```python
from build123d import *

# Parameters (mm, degrees)
F1_DEPTH = 88.9
F3_D     = 19.05
F5_D     = 4.7625


# Not quite as in the source:
# - a feature names something its author has since deleted; it is built from what else it names


with BuildPart() as f1:
    # F0 (on Top) → F1 (new body)
    with BuildSketch(Plane.XY):
        Polygon((10.538799933, 10.6713908286), (-57.7562613184, 10.6713908286), (-65.16550908, 2.3876), (-62.4960911285, 0), (-56.1460911285, 7.0995158286), (8.9414088715, 7.0995158286), (15.2914088715, 0), (17.9537273073, 2.38125), align=None)
    extrude(amount=F1_DEPTH)

    # F3 (through all)
    with Locations(Plane(origin=(0, 10.6713908286, 0), x_dir=(-1, 0, 0), z_dir=(0, 1, 0))):
        with Locations((22.8085911285, 60.325), (23.6087306927, 28.575)):
            Hole(F3_D / 2)

    # F5 (through all)
    with Locations(Plane(origin=(0, 10.6713908286, 0), x_dir=(-1, 0, 0), z_dir=(0, 1, 0))):
        with Locations((-2.5914088715, 82.55), (29.9205911285, 82.55), (29.9205911285, 13.97), (-2.5914088715, 13.97), (48.2085911285, 11.0998), (48.2085911285, 77.7748), (6.9335911285, 77.7748), (6.9335911285, 11.0998)):
            Hole(F5_D / 2)


solid = f1.part
```
Here's how the part is built. I have some questions about the finished solid (model axes, mm). A direction names the side the tool comes from. Coordinates: 2 decimals unless noted, no trailing zeros. Write each loop counter-clockwise with the first axis right and the second up, starting at its lowest first coordinate (ties: lowest second). Pieces come first, ordered by that corner, then holes. Notation, with made-up numbers: (-6, 59) - (44, 59) arc R17 cw to (44, 76) - close; hole circle Ø3 at (73, 75.5). An arc over 180 degrees is marked (long way). One line per item, written item: value.
1) I'm going to push flat-ended pins straight in: P1, Ø5.5, axis at x = 2.59, z = 82.55, coming from the -Y side; P2, Ø3, axis at x = -48.21, z = 11.1, coming from the +Y side; P3, Ø1, axis at y = 6, z = 27, coming from the -X side; P4, Ø1, axis at y = 5.5, z = 49, coming from the +X side. Where does each tip first touch, or does it pass through?
Model answer:
P1: stops at y = 7.1
P2: passes through
P3: stops at x = -62.38
P4: stops at x = 15.61
2) On a 3-axis mill with a long thin cutter (end or side, diameter ignored), from which of +Z, -Z, +X, -X, +Y, -Y can I reach the whole of each face in a straight line? I mean faces 1 (the cylindrical face through (2.075, 8.86, 80.225)), 2 (the flat face through (-24, 7.1, 44)). Say none if no direction works.
Model answer:
face 1: +Y, -Y
face 2: +Z, -Z, -Y
3) Suppose I cut it at D-D on y = 9. State how many separate pieces and enclosed holes the cut face has, and give its area (3 significant figures).
Model answer:
separate pieces: 1
enclosed holes: 10
area: 5,620 mm²
4) Suppose I cut it at C-C on z = 42. Write out the boundary of the cut face in (x, y).
Model answer:
outline: (-65.17, 2.39) - (-62.5, 0) - (-56.15, 7.1) - (8.94, 7.1) - (15.29, 0) - (17.95, 2.38) - (10.54, 10.67) - (-57.76, 10.67) - close
5) I need wall thicknesses on line 1 along Z through (x, y) = (3.5, 8); line 2 along Y through (x, z) = (0, 57); line 3 along X through (y, z) = (6.75, 47). Which ranges of each line are inside material? Lowest first, please.
Model answer:
line 1: z = 0 to 11.77, 16.17 to 80.35, 84.75 to 88.9
line 2: y = 7.1 to 10.67
line 3: x = -61.26 to -56.46, 9.25 to 14.05
6) Suppose I cut it at B-B on x = -48. Write out the boundary of the cut face in (y, z), and give its area (3 significant figures).
Model answer:
outline: (7.1, 0) - (10.67, 0) - (10.67, 8.73) - (7.1, 8.73) - close; (7.1, 13.47) - (10.67, 13.47) - (10.67, 75.4) - (7.1, 75.4) - close; (7.1, 80.15) - (10.67, 80.15) - (10.67, 88.9) - (7.1, 88.9) - close
area: 284 mm²
7) Suppose I cut it at A-A on z = 82.55. Write out the boundary of the cut face in (x, y), and give its area (3 significant figures).
Model answer:
outline: (-65.17, 2.39) - (-62.5, 0) - (-56.15, 7.1) - (-32.3, 7.1) - (-32.3, 10.67) - (-57.76, 10.67) - close; (-27.54, 7.1) - (0.21, 7.1) - (0.21, 10.67) - (-27.54, 10.67) - close; (4.97, 7.1) - (8.94, 7.1) - (15.29, 0) - (17.95, 2.38) - (10.54, 10.67) - (4.97, 10.67) - close
area: 278 mm²
8) We'd pull the mould along X, two halves only. Please class faces 3 (the flat face through (14.298, 6.468, 43.828)), 4 (the flat face through (-63.85, 1.21, 43.83)), 5 (the flat face through (-59.366, 3.5, 43.828)): pulls with the +X half, pulls with the -X half, needs draft (parallel to the pull), parting line crosses it, or undercut.
Model answer:
face 3: pulls with the +X half
face 4: pulls with the -X half
face 5: undercut
